Here's how the part is built. I have some questions about the finished solid (model axes, mm). Face numbers are marked on the shaded views. Give positions to 0.01 mm unless a question says otherwise; leave off trailing zeros. Write each loop counter-clockwise with the first axis right and the second up, starting at its lowest first coordinate (ties: lowest second). Pieces come first, ordered by that corner, then holes. Notation, with made-up numbers: (-26.5, -4) -> (28.5, -4) arc R23 cw to (28.5, 11) -> close; hole circle Ø4 at (84, 0.5). An arc over 180 degrees is marked (long way). Return JSON: item names as keys, results as strings.
from build123d import *

# Parameters (mm, degrees)
F0_W     = 100.076
F0_H     = 88.138
F1_DEPTH = 12.7
F2_R     = 7.91972
F3_DEPTH = 12.701
F4_R     = 3.175
F5_DEPTH = 12.7
F6_R     = 3.175
F7_DEPTH = 12.7


with BuildPart() as f1:
    # F0 (on Top) → F1 (new body)
    with BuildSketch(Plane.XY):
        with Locations((50.038, -44.069)):
            Rectangle(F0_W, F0_H)
    extrude(amount=F1_DEPTH)

    # F2 (on face) → F3 (cut, through all)
    with BuildSketch(Plane.XY.offset(12.7)):
        with Locations((50.038, -38.1)):
            Circle(F2_R)
    extrude(amount=-F3_DEPTH, mode=Mode.SUBTRACT)

    # F4 (on face) → F5 (cut)
    with BuildSketch(Plane.YZ.offset(100.076)):
        with Locations((-81.788, 6.35)):
            Circle(F4_R)
        with Locations((-6.35, 6.35)):
            Circle(F4_R)
    extrude(amount=-F5_DEPTH, mode=Mode.SUBTRACT)

    # F6 (on face) → F7 (cut)
    with BuildSketch(Plane(origin=(0, 0, 0), x_dir=(0, -1, 0), z_dir=(-1, 0, 0))):
        with Locations((6.35, 6.35)):
            Circle(F6_R)
        with Locations((81.788, 6.35)):
            Circle(F6_R)
    extrude(amount=-F7_DEPTH, mode=Mode.SUBTRACT)


solid = f1.part
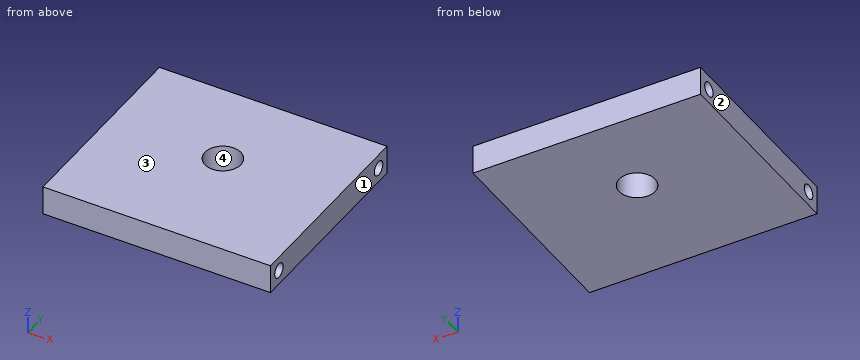
1. Suppose I cut it at C-C, the plane z = 1.5. List the corners of the cut face in (x, y) for me, and give its area (3 significant figures).
Taken from the geometry:
{"outline": "(0, -88.14) -> (100.08, -88.14) -> (100.08, 0) -> (0, 0) -> close; hole circle Ø15.84 at (50.04, -38.1)", "area": "8,620 mm²"}
2. If I drill on line 1 (Y direction, x = 12.5, z = 7.75); line 2 (Z direction, x = 95.75, y = -6.35) (3 decimals); line 3 (X direction, y = -82.5, z = 4.25), over which ranges is the centre line in solid material (lowest first)? Write a range as [from, to].
Taken from the geometry:
{"line 1": "y = [-88.14, -84.64], [-78.94, -9.2], [-3.5, 0]", "line 2": "z = [0, 3.175], [9.525, 12.7]", "line 3": "x = [12.7, 87.38]"}
3. Suppose I cut it at B-B, the plane x = 10.5. List the corners of the cut face in (y, z) for me (3 decimals), and give its area (3 significant figures).
Taken from the geometry:
{"outline": "(-88.138, 0) -> (0, 0) -> (0, 12.7) -> (-88.138, 12.7) -> close; hole circle Ø6.35 at (-81.788, 6.35); hole circle Ø6.35 at (-6.35, 6.35)", "area": "1,060 mm²"}
4. For pin 1 Ø5 at (y, z) = (-82, 6.5) entering from -X; pin 2 Ø5 at (y, z) = (-81.788, 6.35) entering from +X, each with a flat end and sliding along its axis, tell me the tip position at first contact or that it passes through.
Taken from the geometry:
{"pin 1": "stops at x = 12.7", "pin 2": "stops at x = 87.38"}
5. Suppose I cut it at D-D, the plane y = -6.35. List the corners of the cut face in (x, z) for me (3 decimals), and give its area (3 significant figures).
Taken from the geometry:
{"outline": "(0, 0) -> (100.076, 0) -> (100.076, 3.175) -> (87.376, 3.175) -> (87.376, 9.525) -> (100.076, 9.525) -> (100.076, 12.7) -> (0, 12.7) -> (0, 9.525) -> (12.7, 9.525) -> (12.7, 3.175) -> (0, 3.175) -> close", "area": "1,110 mm²"}
6. Suppose I cut it at A-A, the plane y = -38.1. List the corners of the cut face in (x, z) for me.
Taken from the geometry:
{"outline": "(0, 0) -> (42.12, 0) -> (42.12, 12.7) -> (0, 12.7) -> close; (57.96, 0) -> (100.08, 0) -> (100.08, 12.7) -> (57.96, 12.7) -> close"}
7. If we mould it in two halves opening along X, with no side actions, what happens to the marked faces 1, 2, 3 and 4? For each: released by +X, released by -X, zero draft, split by the parting line, or undercut.
Taken from the geometry:
{"face 1": "released by +X", "face 2": "released by -X", "face 3": "zero draft", "face 4": "undercut"}
